from build123d import *

# Parameters (mm, degrees)
BOSS_EXTRUDE1_DEPTH = 15
SKETCH2_W           = 8.7
SKETCH2_H           = 4
CUT_EXTRUDE1_DEPTH  = 15
SKETCH4_R           = 1.1303
CUT_EXTRUDE2_DEPTH  = 15
SKETCH5_R           = 1.215
CUT_EXTRUDE3_DEPTH  = 15
BOSS_EXTRUDE2_DEPTH = 2
FILLET2_R           = 0.5


with BuildPart() as part:
    # Sketch1 → Boss-Extrude1 (new body)
    with BuildSketch(Plane.XY):
        Polygon((0, 0), (0, -6), (-8.7, -6), (-8.7, -11.1), (14.3, -11.1), (14.3, -6), (5.6, -6), (5.6, 0), (3.6, 0), (3.6, -3.541064843), (3.6, -8), (12.3, -8), (12.3, -9.1), (-6.7, -9.1), (-6.7, -8), (2, -8), (2, 0), align=None)
    extrude(amount=BOSS_EXTRUDE1_DEPTH)

    # Sketch2 → Cut-Extrude1 (cut)
    with BuildSketch(Plane(origin=(0, -6, 0), x_dir=(1, 0, 0), z_dir=(0, 1, 0))):
        with Locations((9.95, -13)):
            Rectangle(SKETCH2_W, SKETCH2_H)
    extrude(amount=-CUT_EXTRUDE1_DEPTH, mode=Mode.SUBTRACT)

    # Sketch4 → Cut-Extrude2 (cut)
    with BuildSketch(Plane.ZY):
        with Locations((12.49, -3.148205104)):
            Circle(SKETCH4_R)
        with Locations((6.069694521, -2.53)):
            Circle(SKETCH4_R)
    extrude(amount=-CUT_EXTRUDE2_DEPTH, mode=Mode.SUBTRACT)

    # Sketch5 → Cut-Extrude3 (cut)
    with BuildSketch(Plane(origin=(0, -6, 0), x_dir=(1, 0, 0), z_dir=(0, 1, 0))):
        with Locations((-2.2, -12)):
            Circle(SKETCH5_R)
        with Locations((7.8, -6)):
            Circle(SKETCH5_R)
        with Locations((-2.2, -6)):
            Circle(SKETCH5_R)
    extrude(amount=-CUT_EXTRUDE3_DEPTH, mode=Mode.SUBTRACT)

    # Sketch6 → Boss-Extrude2 (add, symmetric)
    with BuildSketch(Plane(origin=(0, 0, 2), x_dir=(-1, 0, 0), z_dir=(0, 0, -1))):
        Polygon((0, -6), (8.7, -6), (0, 0), align=None)
    boss_extrude2 = extrude(amount=BOSS_EXTRUDE2_DEPTH, both=True)

    # Mirror1: Boss-Extrude2 across plane
    add(boss_extrude2.mirror(Plane(origin=(2.8, 0, 0), x_dir=(0, 0, 1), z_dir=(1, 0, 0))))

    # Fillet2
    fillet2_edges = [part.edges().sort_by_distance(p)[0] for p in [
        (0, -6, 9.5),
        (5.6, -6, 7.5),
    ]]
    fillet(fillet2_edges, radius=FILLET2_R)


solid = part.part
Design review of the part built by this model. Coordinates are the model's own, in mm. A direction names the side the tool comes from. Coordinates: 2 decimals unless noted, no trailing zeros. Write each loop counter-clockwise with the first axis right and the second up, starting at its lowest first coordinate (ties: lowest second). Pieces come first, ordered by that corner, then holes. Notation, with made-up numbers: (43, -14.75) -> (79, -14.75) arc R13 cw to (79, -7.75) -> close; hole circle Ø5 at (-4, 36.25). An arc over 180 degrees is marked (long way). Write each question's results on one line, items separated by ' | '. Start each with the question number.
(1) Take a section at B-B on x = 0.5. Write out the cut boundary in (y, z).
(2) Take a section at C-C on z = 2.5. Write out the cut boundary in (x, y), and give its area (3 significant figures).
(3) Clearance check with flat-ended pins moving along their axes: P1, Ø1.4, axis at y = -3.15, z = 12.49, coming from the +X side; P2, Ø3, axis at x = 7.8, z = 6, coming from the +Y side; P3, Ø6.5, axis at y = -2, z = 7.5, coming from the -X side; P4, Ø2.5, axis at y = -2.53, z = 6.07, coming from the +X side. State where each tip first meets the part, or that it passes through.
(4) For line 1 along Z through (x, y) = (-2.2, -6.75) (3 decimals); line 2 along X through (y, z) = (-7.3, 12) (3 decimals); line 3 along Y through (x, z) = (-3, 8.25), list the stretches that pass through material, from the lowest coordinate up. Write a range as from..to.
(5) Tool access review of faces 4 (the face through (-2.4, -7, 4.8)), 5 (the face through (5.6, -3, 9)), 6 (the face through (2, -4, 7)), 7 (the face through (5.6, -10, 13)), 8 (the face through (7.9, -8, 7.4)): name each direction out of +Z, -Z, +X, -X, +Y, -Y from which nothing blocks a thin tool from reaching the whole face with its end or side.
(6) The part is to be moulded in two halves that separate along Y. For faces 1 (the face through (3, -9.1, 7)), 2 (the face through (10, -6, 7)), 3 (the face through (-2.463, -10.086, 13.186)), say which applies: pulls with the +Y half, pulls with the -Y half, needs draft (parallel to the pull), parting line crosses it, or undercut.
(7) Take a section at D-D on y = -9.75. Write out the cut boundary in (x, z) (3 decimals), and give its area (3 significant figures).
(8) Take a section at A-A on y = -7.5. Write out the cut boundary in (x, z) (3 decimals).
Results found:
1) outline: (-11.1, 0) -> (-9.1, 0) -> (-9.1, 15) -> (-11.1, 15) -> close; (-8, 0) -> (0, 0) -> (0, 15) -> (-8, 15) -> close; hole circle Ø2.26 at (-3.15, 12.49); hole circle Ø2.26 at (-2.53, 6.07)
2) outline: (-8.7, -11.1) -> (14.3, -11.1) -> (14.3, -6) -> (5.6, 0) -> (3.6, 0) -> (3.6, -8) -> (12.3, -8) -> (12.3, -9.1) -> (-6.7, -9.1) -> (-6.7, -8) -> (2, -8) -> (2, 0) -> (0, 0) -> (-8.7, -6) -> close | area: 169 mm2
3) P1: passes through | P2: stops at y = -6 | P3: stops at x = 0 | P4: stops at x = 5.6
4) line 1: z = 0..4.785, 7.215..10.785, 13.215..15 | line 2: x = -8.7..-3.415, -0.985..2, 3.6..5.6 | line 3: y = -11.1..-9.1, -8..-6
5) face 4: +Y, -Y | face 5: +Z, +X, +Y | face 6: +Z, -Z, +Y | face 7: +Z, +X, +Y, -Y | face 8: +Z, -Z
6) face 1: undercut | face 2: pulls with the +Y half | face 3: needs draft
7) outline: (-8.7, 0) -> (14.3, 0) -> (14.3, 11) -> (5.6, 11) -> (5.6, 15) -> (-8.7, 15) -> close; hole circle Ø2.43 at (-2.2, 6); hole circle Ø2.43 at (-2.2, 12); hole circle Ø2.43 at (7.8, 6) | area: 296 mm2
8) outline: (-8.7, 0) -> (2, 0) -> (2, 15) -> (-8.7, 15) -> close; (3.6, 0) -> (14.3, 0) -> (14.3, 11) -> (5.6, 11) -> (5.6, 15) -> (3.6, 15) -> close; hole circle Ø2.43 at (-2.2, 6); hole circle Ø2.43 at (-2.2, 12); hole circle Ø2.43 at (7.8, 6)
